For this review, use the dimensioned drawing (mm, ordinates from the lowest corner) and the shaded views. A direction names the side the tool comes from. Round coordinates to 2 decimals unless told otherwise and drop trailing zeros. Write each loop counter-clockwise with the first axis right and the second up, starting at its lowest first coordinate (ties: lowest second). Pieces come first, ordered by that corner, then holes. Notation, with made-up numbers: M -16,-32.75 L 11,-32.75 A17 ccw 11,-18.75 Z; hole C 26,-13.5 d9. An arc over 180 degrees is marked long. Use CSV: the item, a comma, the result in double quotes.
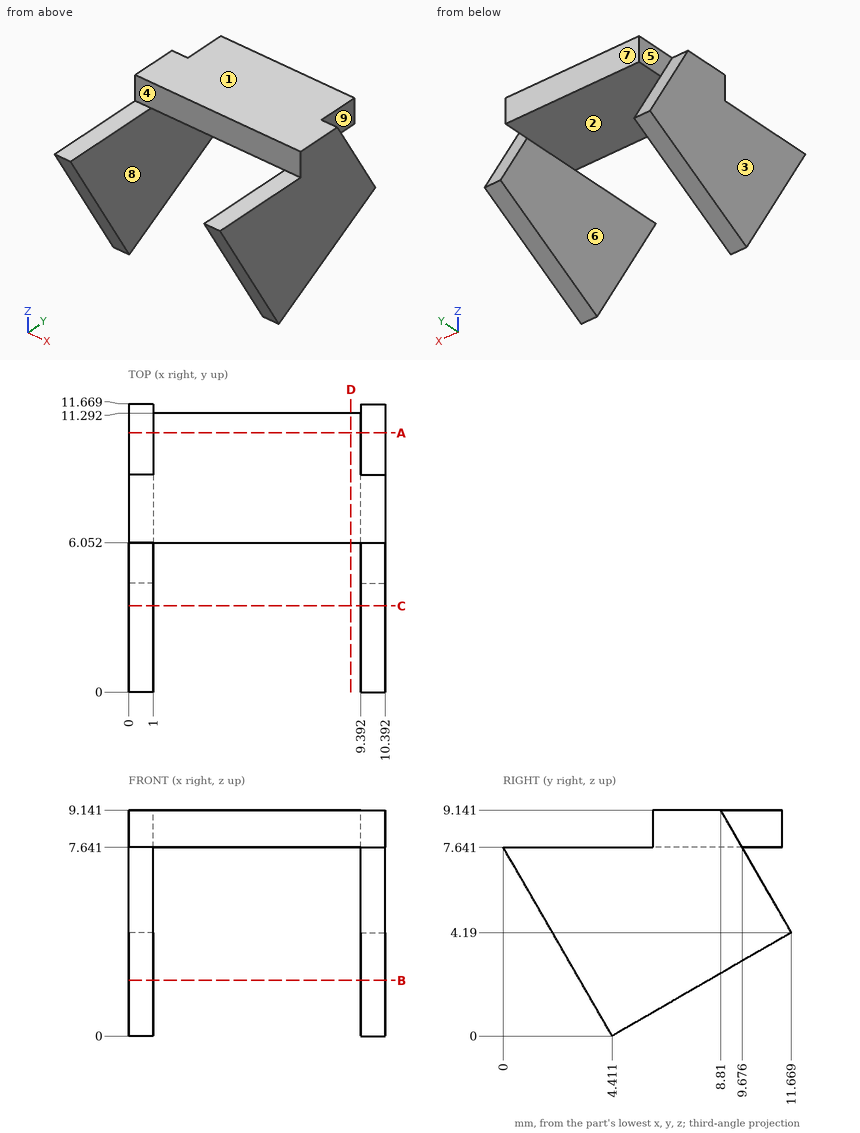
1) Add section B-B on z = 2.25. Write out the cut boundary in (x, y), then the cut area to 3 significant figures.
Answers:
outline,"M 0,3.11 L 1,3.11 L 1,8.31 L 0,8.31 Z; M 9.39,3.11 L 10.39,3.11 L 10.39,8.31 L 9.39,8.31 Z"
area,"10.4 mm²"
2) The part is to be moulded in two halves that separate along X. For the marked faces 6, 7, 8 and 9, say which applies: released by +X, released by -X, zero draft, split by the parting line, or undercut.
Answers:
face 6,"undercut"
face 7,"zero draft"
face 8,"undercut"
face 9,"released by +X"
3) Add section D-D on x = 9. Write out the cut boundary in (y, z).
Answers:
outline,"M 6.05,7.64 L 11.29,7.64 L 11.29,9.14 L 6.05,9.14 Z"
4) Machinability: for the marked faces 1, 2, 3, 4 and 5, which of the approach directions +Z, -Z, +X, -X, +Y, -Y give a long, thin tool a straight path to every point of the face, cutting with its end or side? Answer none if there is none.
Answers:
face 1,"+Z, +X, -X, +Y, -Y"
face 2,"-Z, +Y, -Y"
face 3,"+Z, -Z, -X, +Y, -Y"
face 4,"+Z, +X, -X, -Y"
face 5,"+Z, -X, +Y"
5) Wall thickness on line 1 along X through (y, z) = (9.75, 4.25); line 2 along Z through (x, y) = (7, 7.25); line 3 along Y through (x, z) = (7.5, 7.75): over which ranges is each line inside the solid? List them lowest first. Write a range as [from, to].
Answers:
line 1,"[0, 1], [9.39, 10.39]"
line 2,"[7.64, 9.14]"
line 3,"[6.05, 11.29]"
6) Add section C-C on y = 3.5. Write out the cut boundary in (x, z), then the cut area to 3 significant figures.
Answers:
outline,"M 0,1.58 L 1,1.58 L 1,7.64 L 0,7.64 Z; M 9.39,1.58 L 10.39,1.58 L 10.39,7.64 L 9.39,7.64 Z"
area,"12.1 mm²"
7) For pin 1 Ø2 at (y, z) = (6.5, 4) entering from -X; pin 2 Ø1 at (x, z) = (2.5, 2.5) entering from +Y; pin 3 Ø1.5 at (x, y) = (6.5, 8.5) entering from -Z; pin 4 Ø0.8 at (x, y) = (10, 4) entering from +Z, all flat-tipped, find the tip position at first contact; note any pin that passes through.
Answers:
pin 1,"x = 0"
pin 2,"through"
pin 3,"z = 7.64"
pin 4,"z = 7.64"
8) Add section A-A on y = 10.5. Write out the cut boundary in (x, z) (1 decimal), then the cut area to 3 significant figures.
Answers:
outline,"M 0,3.5 L 1,3.5 L 1,6.2 L 0,6.2 Z; M 1,7.6 L 9.4,7.6 L 9.4,9.1 L 1,9.1 Z; M 9.4,3.5 L 10.4,3.5 L 10.4,6.2 L 9.4,6.2 Z"
area,"18.0 mm²"
